Check sheet for the modelled part. Datum: model origin and axes. Units: mm. Round coordinates to 2 decimals unless told otherwise and drop trailing zeros. Order: outer loops, then holes, each group sorted by start corner. A loop starts at its lowest first (then second) coordinate and runs counter-clockwise, first axis right, second up.
Autodesk Fusion 360 part; units mm, degrees
sketch "Esquisse1" plane through (0, 0, 0) normal (0, 1, 0) x (1, 0, 0)
  line L0 (11.547, -20) -> (23.094, 0)
  line L1 (23.094, 0) -> (11.547, 20)
  line L2 (11.547, 20) -> (-11.547, 20)
  line L3 (-11.547, 20) -> (-23.094, 0)
  line L4 (-23.094, 0) -> (-11.547, -20)
  line L5 (-11.547, -20) -> (11.547, -20)
  dimension "d1" = 20
extrude "Extrusion1" add sketch "Esquisse1" along normal blind 95
sketch "Esquisse3" plane through (0, 0, 0) normal (0, 0, 1) x (1, 0, 0)
  line L0 (11.547, 95) -> (-11.547, 95)
  line L1 (-2.8927, 95) -> (-23.094, 45)
  line L2 (-23.094, 45) -> (-23.094, 95)
  line L3 (-23.094, 95) -> (-2.8927, 95)
  line L4 (-23.094, 0) -> (-23.094, 95)
  point P0 (0, 95)
  dimension "d8" = 50
  dimension "d9" = 22
revolve "Révolution1" cut sketch "Esquisse3" angle 360 about axis through (0, 1.75, 0) along (0, 1, 0)
extrude "Extrusion2" cut 1 faces at (0.2146, 95, -0.8551) along direction (0, -1, 0) blind 130
hole "Perçage1" at (0, 0, 0) direction (0, 1, 0) diameter 30 depth 40 tip angle 180
Item 1: Release check for a two-part mould opening along Z. For faces 1 (the flat face through (3.1, 40, 0.2)), 2 (the cylindrical face through (-0.66, 20.28, 14.985)), 3 (the flat face through (-17.4, 25.96, 9.86)), 4 (the flat face through (0, 26, -20)) record: released by +Z, released by -Z, zero draft, split by the parting line, or undercut.
Answer:
face 1: undercut
face 2: undercut
face 3: released by +Z
face 4: released by -Z
Item 2: Go/stop test with flat-tipped pins: P1, Ø18, axis at x = 0, z = 0, coming from the -Y side; P2, Ø10, axis at y = 79, z = -12, coming from the +X side; P3, Ø8, axis at x = -16, z = 9.5, coming from the -Y side; P4, Ø5, axis at y = 25.5, z = 2, coming from the +X side. Record where each tip stops, or that it passes through.
Answer:
P1: stops at y = 40
P2: stops at x = 6.98
P3: stops at y = 0
P4: stops at x = 23.09
Item 3: Sectioned sample at B-B (y = 36). Record the cut outline in (x, z), and give its area (3 significant figures).
Answer:
outline: (-23.09, 0) - (-11.55, -20) - (11.55, -20) - (23.09, 0) - (11.55, 20) - (-11.55, 20) - close; hole circle Ø30 at (0, 0)
area: 679 mm2
Item 4: Sectioned sample at A-A (x = 0). Record the cut outline in (y, z), and give its area (3 significant figures).
Answer:
outline: (0, -20) - (52.66, -20) - (95, -2.89) - (40, -2.89) - (40, -15) - (0, -15) - close; (0, 15) - (40, 15) - (40, 2.89) - (95, 2.89) - (52.66, 20) - (0, 20) - close
area: 1,560 mm2
Item 5: Scan lines: line 1 along Z through (x, y) = (0, 8.5); line 2 along X through (y, z) = (19.5, 0); line 3 along Z through (x, y) = (-8.5, 7.5). Record each from-to range of solid material in increasing order.
Answer:
line 1: z = -20 to -15, 15 to 20
line 2: x = -23.09 to -15, 15 to 23.09
line 3: z = -20 to -12.36, 12.36 to 20
